Model file for the job. Use its own axes, mm. A direction names the side the tool comes from. Give positions to 0.01 mm unless a question says otherwise; leave off trailing zeros. Loops run counter-clockwise (first coordinate to the right, second up) from the corner with the lowest first, then second, coordinate; pieces in that order, holes last. Notation, with made-up numbers: (-12, 75) - (-1, 75) arc R22 ccw to (-1, 99) - close; hole circle Ø6 at (81.25, -7). An arc over 180 degrees is marked (long way). Use a Markdown table: item, result.
from build123d import *

# Parameters (mm, degrees)
SKETCH2_R                = 13.85
SKETCH2_R_2              = 4
SKETCH2_R_3              = 1.5
BOSS_EXTRUDE1_DEPTH      = 5
SKETCH3_R                = 4
BOSS_EXTRUDE2_DEPTH      = 17
BOSS_EXTRUDE2_DEPTH_BACK = 5
CUT_EXTRUDE1_DEPTH       = 10


with BuildPart() as part:
    # Sketch2 → Boss-Extrude1 (new body)
    with BuildSketch(Plane.XY):
        Circle(SKETCH2_R)
        Circle(SKETCH2_R_2, mode=Mode.SUBTRACT)
        with Locations((0, 8)):
            Circle(SKETCH2_R_3, mode=Mode.SUBTRACT)
        with Locations((-8, 0)):
            Circle(SKETCH2_R_3, mode=Mode.SUBTRACT)
        with Locations((8, 0)):
            Circle(SKETCH2_R_3, mode=Mode.SUBTRACT)
        with Locations((0, -8)):
            Circle(SKETCH2_R_3, mode=Mode.SUBTRACT)
    extrude(amount=BOSS_EXTRUDE1_DEPTH)

    # Sketch3 → Boss-Extrude2 (add, two sides)
    with BuildSketch(Plane.XY.offset(5)) as boss_extrude2_sk:
        Circle(SKETCH3_R)
    extrude(amount=BOSS_EXTRUDE2_DEPTH)
    extrude(boss_extrude2_sk.sketch, amount=-BOSS_EXTRUDE2_DEPTH_BACK)

    # Sketch4 → Cut-Extrude1 (cut)
    with BuildSketch(Plane.XY.offset(22)):
        with BuildLine():
            Line((-2.645751311, 3), (2.645751311, 3))
            ThreePointArc((2.645751311, 3), (0, 4), (-2.645751311, 3))
        make_face()
    extrude(amount=-CUT_EXTRUDE1_DEPTH, mode=Mode.SUBTRACT)


solid = part.part
(1) Mould opens along X. For faces 1 (the cylindrical face through (13.21, 4.16, 2.46)), 2 (the flat face through (0, 0, 0)), 3 (the cylindrical face through (-0.325, 6.536, 2.465)) say: pulls with the +X half, pulls with the -X half, needs draft (parallel to the pull), parting line crosses it, or undercut.
Computed:
| item | result |
|---|---|
| face 1 | parting line crosses it |
| face 2 | needs draft |
| face 3 | undercut |
(2) 3-axis set-ups, long thin cutter, end or side, ignore diameter. For faces 4 (the flat face through (0, 3.4, 12)), 5 (the cylindrical face through (-0.867, -3.905, 13.381)), 6 (the cylindrical face through (-9.5, 0.07, 2.46)): which of +Z, -Z, +X, -X, +Y, -Y reach the whole face in a straight line?
Computed:
| item | result |
|---|---|
| face 4 | +Z, +X, -X, +Y |
| face 5 | +Z |
| face 6 | +Z, -Z |
(3) Slice it at B-B, the plane x = 8. Write the cut outline in (y, z), plus the area to 3 significant figures.
Computed:
| item | result |
|---|---|
| outline | (-11.31, 0) - (-1.5, 0) - (-1.5, 5) - (-11.31, 5) - close; (1.5, 0) - (11.31, 0) - (11.31, 5) - (1.5, 5) - close |
| area | 98.1 mm² |
(4) Pin check, flat tips, straight feed: P1, Ø1.8, axis at x = 0, y = -8, coming from the -Z side; P2, Ø8, axis at x = 9, z = 4.5, coming from the -Y side; P3, Ø8.5, axis at x = -3, y = 4, coming from the +Z side; P4, Ø2, axis at x = 10, z = 5, coming from the -Y side. Stop position of each tip, or through.
Computed:
| item | result |
|---|---|
| P1 | through |
| P2 | y = -12.92 |
| P3 | z = 22 |
| P4 | y = -10.53 |
(5) Drill centre lines: probe 1 along Y at (x, z) = (0, 1.95); probe 2 along Y at (x, z) = (0.5, 1.5); probe 3 along Z at (x, y) = (4.5, 5). Where is each one in solid material? Low to high. Write a range as [from, to].
Computed:
| item | result |
|---|---|
| probe 1 | [-13.85, -9.5], [-6.5, 6.5], [9.5, 13.85] |
| probe 2 | [-13.84, -9.41], [-6.59, 6.59], [9.41, 13.84] |
| probe 3 | [0, 5] |
(6) Slice it at A-A, the plane y = 0. Write the cut outline in (x, z).
Computed:
| item | result |
|---|---|
| outline | (-13.85, 0) - (-9.5, 0) - (-9.5, 5) - (-13.85, 5) - close; (-6.5, 0) - (6.5, 0) - (6.5, 5) - (4, 5) - (4, 22) - (-4, 22) - (-4, 5) - (-6.5, 5) - close; (9.5, 0) - (13.85, 0) - (13.85, 5) - (9.5, 5) - close |
(7) Slice it at C-C, the plane x = 0. Write the cut outline in (y, z).
Computed:
| item | result |
|---|---|
| outline | (-13.85, 0) - (-9.5, 0) - (-9.5, 5) - (-13.85, 5) - close; (-6.5, 0) - (6.5, 0) - (6.5, 5) - (4, 5) - (4, 12) - (3, 12) - (3, 22) - (-4, 22) - (-4, 5) - (-6.5, 5) - close; (9.5, 0) - (13.85, 0) - (13.85, 5) - (9.5, 5) - close |
